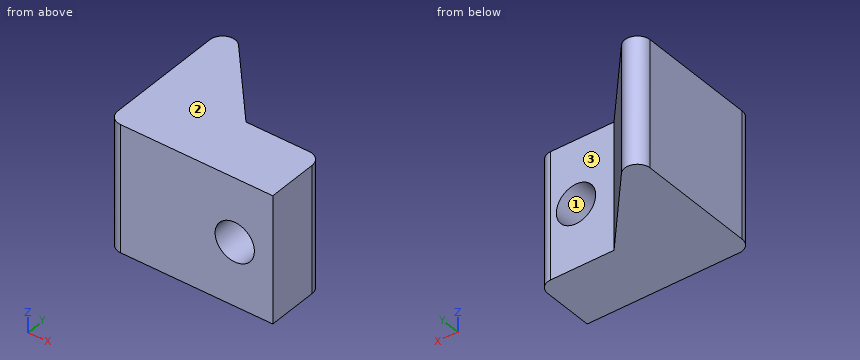
```python
from build123d import *

# Parameters (mm, degrees)
BOSS_EXTRUDE1_DEPTH = 5
SKETCH2_R           = 1.55
CUT_EXTRUDE1_DEPTH  = 10


with BuildPart() as part:
    # Sketch1 → Boss-Extrude1 (new, symmetric)
    with BuildSketch(Plane.XY):
        with BuildLine():
            Line((1, 0), (13, 0))
            Line((13, 0), (13, 4))
            ThreePointArc((13, 4), (12.707106781, 4.707106781), (12, 5))
            Line((12, 5), (7, 5))
            Line((7, 5), (1.752576695, 10.997055206))
            ThreePointArc((1.752576695, 10.997055206), (0.648273327, 11.274653342), (0, 10.338550598))
            Line((0, 10.338550598), (0, 1))
            ThreePointArc((0, 1), (0.292893219, 0.292893219), (1, 0))
        make_face()
    extrude(amount=BOSS_EXTRUDE1_DEPTH, both=True)

    # Sketch2 → Cut-Extrude1 (cut)
    with BuildSketch(Plane.XZ):
        with Locations(Location((10, 0, 0), (0, 0, 270))):
            Circle(SKETCH2_R)
    extrude(amount=-CUT_EXTRUDE1_DEPTH, mode=Mode.SUBTRACT)


solid = part.part
```
For this review, take the finished solid that the model builds, in its own axes (mm). Face numbers are marked on the shaded views. Round coordinates to 2 decimals unless told otherwise and drop trailing zeros. Write each loop counter-clockwise with the first axis right and the second up, starting at its lowest first coordinate (ties: lowest second). Pieces come first, ordered by that corner, then holes.
1) Take a section at B-B on x = 10.75. Give the boundary of the cut face in (y, z).
Answer below:
outline: (0, -5) - (5, -5) - (5, -1.36) - (0, -1.36) - close; (0, 1.36) - (5, 1.36) - (5, 5) - (0, 5) - close
2) For line 1 along X through (y, z) = (2.9, 0); line 2 along Y through (x, z) = (8.75, 4.5); line 3 along Z through (x, y) = (9.75, 1.75), list the stretches that pass through material, from the lowest coordinate up.
Answer below:
line 1: x = 0 to 8.45, 11.55 to 13
line 2: y = 0 to 5
line 3: z = -5 to -1.53, 1.53 to 5
3) Take a section at A-A on z = 0. Give the boundary of the cut face in (x, y), then the cut area to 3 significant figures.
Answer below:
outline: (0, 1) arc R1 ccw to (1, 0) - (8.45, 0) - (8.45, 5) - (7, 5) - (1.75, 11) arc R1 ccw to (0, 10.34) - close; (11.55, 0) - (13, 0) - (13, 4) arc R1 ccw to (12, 5) - (11.55, 5) - close
area: 75.6 mm2
4) Mouldability with a two-part tool opening along Z and no side actions: class the marked faces 1, 2 and 3 as +Z half, -Z half, draft (parallel to the pull), parting line (faces both ways), or undercut.
Answer below:
face 1: undercut
face 2: +Z half
face 3: draft
5) Take a section at C-C on z = -3.75. Give the boundary of the cut face in (x, y), then the cut area to 3 significant figures.
Answer below:
outline: (0, 1) arc R1 ccw to (1, 0) - (13, 0) - (13, 4) arc R1 ccw to (12, 5) - (7, 5) - (1.75, 11) arc R1 ccw to (0, 10.34) - close
area: 91.1 mm2
6) Insertion check: pin 1 Ø3 at (x, z) = (10, 0) entering from +Y; pin 2 Ø3 at (y, z) = (5, 1) entering from +X; pin 3 Ø2.5 at (x, z) = (9, -1) entering from +Y; pin 4 Ø5 at (y, z) = (10, 0.5) entering from +X. Each pin has a flat end and moves straight along its axis. Give the tip position at first contact, or say it passes through.
Answer below:
pin 1: passes through
pin 2: stops at x = 13
pin 3: stops at y = 5
pin 4: stops at x = 4.81
7) Take a section at D-D on z = 1. Give the boundary of the cut face in (x, y).
Answer below:
outline: (0, 1) arc R1 ccw to (1, 0) - (8.82, 0) - (8.82, 5) - (7, 5) - (1.75, 11) arc R1 ccw to (0, 10.34) - close; (11.18, 0) - (13, 0) - (13, 4) arc R1 ccw to (12, 5) - (11.18, 5) - close
